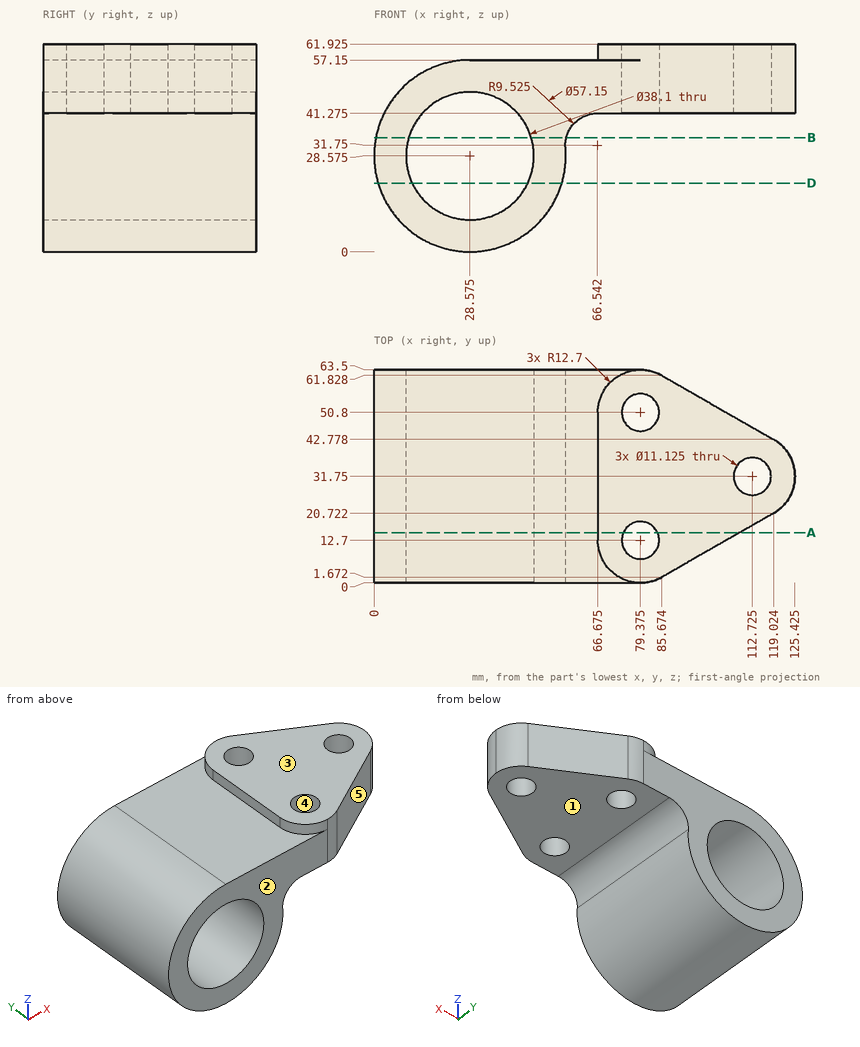
Geometry: see drawing. Coordinates: mm, zero at the bounding-box minimum. A direction names the side the tool comes from. Round coordinates to 2 decimals unless told otherwise and drop trailing zeros. Write each loop counter-clockwise with the first axis right and the second up, starting at its lowest first coordinate (ties: lowest second). Pieces come first, ordered by that corner, then holes.
1) Draft query along Y for the marked faces 3, 4 and 5. Return one class per face: pulls with the +Y half, pulls with the -Y half, needs draft (parallel to the pull), parting line crosses it, or undercut.
2) Contact query for flat-ended pins moving along their axis: P1, Ø2, axis at y = 56, z = 50.5, coming from the +X side (1 decimal); P2, Ø17.5, axis at x = 85.5, y = 30, coming from the -Z side (3 decimals); P3, Ø1.5, axis at y = 44.5, z = 16, coming from the +X side. Output: stop coordinate, or through.
3) Cut plane D-D (z = 20.5). Return the cut outline in (x, y) (1 decimal), then the cut area to 3 significant figures.
4) Reachability of the marked faces 1 and 2 from +Z, -Z, +X, -X, +Y, -Y: full face, straight path, thin tool, end or side. Return the list, or none.
5) Ray query, L1, parallel to Y at x = 79, z = 42.5; L2, parallel to Z at x = 88, y = 36.5 (1 decimal); L3, parallel to X at y = 29.5, z = 29. Return the intervals inside material, ascending.
6) Cut plane A-A (y = 15). Count the separate pieces of the cut face and the enclosed holes in it, then the cut area to 3 significant figures.
7) Cut plane B-B (z = 34). Return the cut outline in (x, y).
Geometry says:
1. face 3: needs draft
1. face 4: undercut
1. face 5: pulls with the -Y half
2. P1: stops at x = 97.6
2. P2: stops at z = 41.275
2. P3: stops at x = 54.59
3. outline: (1.2, 0) - (11.3, 0) - (11.3, 63.5) - (1.2, 63.5) - close; (45.8, 0) - (56, 0) - (56, 63.5) - (45.8, 63.5) - close
3. area: 1,290 mm2
4. face 1: -Z, +X, +Y, -Y
4. face 2: +Z, -Z, +X, -X, -Y
5. L1: y = 0 to 7.15, 18.25 to 45.25, 56.35 to 63.5
5. L2: z = 41.3 to 61.9
5. L3: x = 0 to 9.53, 47.62 to 57.15
6. separate pieces: 2
6. enclosed holes: 1
6. area: 2,430 mm2
7. outline: (0.52, 0) - (10.31, 0) - (10.31, 63.5) - (0.52, 63.5) - close; (46.84, 0) - (57.29, 0) - (57.29, 63.5) - (46.84, 63.5) - close
